The model under review builds one solid part; all positions refer to its coordinate system, in mm. A direction names the side the tool comes from. Round coordinates to 2 decimals unless told otherwise and drop trailing zeros. Write each loop counter-clockwise with the first axis right and the second up, starting at its lowest first coordinate (ties: lowest second). Pieces come first, ordered by that corner, then holes. Notation, with made-up numbers: M 30.5,69 L 48.5,69 A13 ccw 48.5,73 Z; hole C 32.25,3 d7. An arc over 180 degrees is marked long. One line per item, written item: value. Start each with the question number.
1) Take a section at D-D, the plane z = -28.5. Write out the cut boundary in (x, y), and give its area (3 significant figures).
2) Take a section at C-C, the plane y = 13.5. Write out the cut boundary in (x, z), and give its area (3 significant figures).
3) Wall thickness on probe 1 along Y at (x, z) = (-10, -21); probe 2 along Y at (x, z) = (-10, 1.1); probe 3 along Z at (x, y) = (15, 19): over which ranges is each line inside the solid? List them lowest first.
4) Mouldability with a two-part tool opening along Z and no side actions: class faces 3 (the face through (11.066, -11.74, -48.523)), 4 (the face through (-17.08, -11.74, -7.01)), 5 (the face through (0, -11, -51)) as +Z half, -Z half, draft (parallel to the pull), parting line (faces both ways), or undercut.
5) For P1, Ø11, axis at x = -1.5, y = 19, coming from the -Z side; P2, Ø2.5, axis at x = -10, z = -6.5, coming from the +Y side; P3, Ø1.5, axis at x = -3, z = -10, coming from the +Y side; P4, Ø4, axis at x = 10, y = 22.5, coming from the +Z side, all flat-tipped, find the tip position at first contact; note any pin that passes through.
6) Take a section at B-B, the plane y = 2.5. Write out the cut boundary in (x, z), and give its area (3 significant figures).
7) Take a section at A-A, the plane x = 0. Write out the cut boundary in (y, z).
8) Tool access review of faces 1 (the face through (0, 6, 1.5)), 2 (the face through (0, 6, 0)): name each direction out of +Z, -Z, +X, -X, +Y, -Y from which nothing blocks a thin tool from reaching the whole face with its end or side.
from build123d import *

# Parameters (mm, degrees)
SKETCH2_R                    = 1.5
BOSS_EXTRUDE1_DEPTH          = 1.5
EDGE_FLANGE1_STRIP_W         = 9
EDGE_FLANGE1_STRIP_H         = 1.5
EDGE_FLANGE1_STRIP_CUT_DEPTH = 36
EDGE_FLANGE1_DEPTH           = 36
CUT_EXTRUDE1_DEPTH           = 1.5
FILLET1_R                    = 10
SKETCH12_R                   = 1.5
CUT_EXTRUDE2_DEPTH           = 15


# Sheet-metal steps are written as plain solids
with BuildPart() as part:
    # Sketch2 → Boss-Extrude1 (new body)
    with BuildSketch(Plane.XY):
        with BuildLine():
            ThreePointArc((18, 12.5), (0, 30.5), (-18, 12.5))
            Line((-18, 12.5), (-18, -12.5))
            Line((-18, -12.5), (18, -12.5))
            Line((18, -12.5), (18, 12.5))
        make_face()
        with Locations((-10, 2.5)):
            Circle(SKETCH2_R, mode=Mode.SUBTRACT)
        with BuildLine():
            ThreePointArc((-3.535533906, 16.035533906), (0, 17.5), (3.535533906, 16.035533906))
            ThreePointArc((3.535533906, 16.035533906), (5, 12.5), (3.535533906, 8.964466094))
            ThreePointArc((3.535533906, 8.964466094), (0, 7.5), (-3.535533906, 8.964466094))
            ThreePointArc((-3.535533906, 8.964466094), (-5, 12.5), (-3.535533906, 16.035533906))
        make_face(mode=Mode.SUBTRACT)
        with Locations((10, 2.5)):
            Circle(SKETCH2_R, mode=Mode.SUBTRACT)
        with Locations((-10, 22.5)):
            Circle(SKETCH2_R, mode=Mode.SUBTRACT)
        with Locations((10, 22.5)):
            Circle(SKETCH2_R, mode=Mode.SUBTRACT)
    extrude(amount=BOSS_EXTRUDE1_DEPTH)

    # Edge-Flange1 strip (across the edge) → Edge-Flange1 strip cut (cut)
    with BuildSketch(Plane(origin=(18, -12.5, 0), x_dir=(0, 1, 0), z_dir=(-1, 0, 0))):
        with Locations((-1.5, -0.75)):
            Rectangle(EDGE_FLANGE1_STRIP_W, EDGE_FLANGE1_STRIP_H)
    extrude(amount=EDGE_FLANGE1_STRIP_CUT_DEPTH, mode=Mode.SUBTRACT)

    # Edge-Flange1 section (across the edge) → Edge-Flange1 (add)
    with BuildSketch(Plane(origin=(18, -12.5, 0), x_dir=(0, 1, 0), z_dir=(-1, 0, 0))):
        with BuildLine():
            Line((0, 1.5), (0, 98.5))
            Line((0, 98.5), (1.5, 98.5))
            Line((1.5, 98.5), (1.5, 1.5))
            ThreePointArc((1.5, 1.5), (1.939339828, 0.439339828), (3, 0))
            Line((3, 0), (3, -1.5))
            ThreePointArc((3, -1.5), (0.878679656, -0.621320344), (0, 1.5))
        make_face()
    extrude(amount=EDGE_FLANGE1_DEPTH)

    # Sketch11 → Cut-Extrude1 (cut)
    with BuildSketch(Plane(origin=(0, -11, 0), x_dir=(1, 0, 0), z_dir=(0, 1, 0))):
        with BuildLine():
            Line((-18, 98.5), (-18, 1.5))
            Line((-18, 1.5), (-16, 13.5))
            Line((-16, 13.5), (-16, 93.5))
            ThreePointArc((-16, 93.5), (-14.535533906, 97.035533906), (-11, 98.5))
            Line((-11, 98.5), (-18, 98.5))
        make_face()
        with BuildLine():
            Line((16, 13.5), (18, 1.5))
            Line((18, 1.5), (18, 98.5))
            Line((18, 98.5), (11, 98.5))
            ThreePointArc((11, 98.5), (14.535533906, 97.035533906), (16, 93.5))
            Line((16, 93.5), (16, 13.5))
        make_face()
    extrude(amount=-CUT_EXTRUDE1_DEPTH, mode=Mode.SUBTRACT)

    # Fillet1
    fillet1_edges = [part.edges().sort_by_distance(p)[0] for p in [
        (-16, -11.75, -13.5),
        (16, -11.75, -13.5),
    ]]
    fillet(fillet1_edges, radius=FILLET1_R)

    # Sketch12 → Cut-Extrude2 (cut)
    with BuildSketch(Plane(origin=(0, -11, 0), x_dir=(1, 0, 0), z_dir=(0, 1, 0))):
        with Locations(Location((-10, 6.5, 0), (0, 0, 270))):
            Circle(SKETCH12_R)
        with Locations(Location((-11, 31.5, 0), (0, 0, 270))):
            Circle(SKETCH12_R)
        with Locations(Location((-11, 47.024174696, 0), (0, 0, 270))):
            Circle(SKETCH12_R)
        with Locations(Location((-11, 62.024174696, 0), (0, 0, 270))):
            Circle(SKETCH12_R)
        with Locations(Location((-11, 77.024174696, 0), (0, 0, 270))):
            Circle(SKETCH12_R)
        with Locations(Location((-11, 92.024174696, 0), (0, 0, 270))):
            Circle(SKETCH12_R)
        with Locations(Location((11, 92.024174696, 0), (0, 0, 270))):
            Circle(SKETCH12_R)
        with Locations(Location((11, 77.024174696, 0), (0, 0, 270))):
            Circle(SKETCH12_R)
        with Locations(Location((11, 62.024174696, 0), (0, 0, 270))):
            Circle(SKETCH12_R)
        with Locations(Location((11, 47.024174696, 0), (0, 0, 270))):
            Circle(SKETCH12_R)
        with Locations(Location((11, 31.5, 0), (0, 0, 270))):
            Circle(SKETCH12_R)
        with Locations(Location((10, 6.5, 0), (0, 0, 270))):
            Circle(SKETCH12_R)
    extrude(amount=-CUT_EXTRUDE2_DEPTH, mode=Mode.SUBTRACT)


solid = part.part
Checked values:
1. outline: M -16,-12.5 L 16,-12.5 L 16,-11 L -16,-11 Z
1. area: 48.0 mm2
2. outline: M -17.97,0 L -4.9,0 L -4.9,1.5 L -17.97,1.5 Z; M 4.9,0 L 17.97,0 L 17.97,1.5 L 4.9,1.5 Z
2. area: 39.2 mm2
3. probe 1: y = -12.5 to -11
3. probe 2: y = -11 to 1, 4 to 21, 24 to 27.47
3. probe 3: z = 0 to 1.5
4. face 3: undercut
4. face 4: -Z half
4. face 5: draft
5. P1: stops at z = 0
5. P2: passes through
5. P3: stops at y = -11
5. P4: stops at z = 1.5
6. outline: M -18,0 L -11.5,0 L -11.5,1.5 L -18,1.5 Z; M -8.5,0 L 8.5,0 L 8.5,1.5 L -8.5,1.5 Z; M 11.5,0 L 18,0 L 18,1.5 L 11.5,1.5 Z
6. area: 45.0 mm2
7. outline: M -12.5,-98.5 L -11,-98.5 L -11,-1.5 A1.5 cw -9.5,0 L 7.5,0 L 7.5,1.5 L -9.5,1.5 A3 ccw -12.5,-1.5 Z; M 17.5,0 L 30.5,0 L 30.5,1.5 L 17.5,1.5 Z
8. face 1: +Z, +X, -X, +Y, -Y
8. face 2: -Z, +X, -X, +Y
